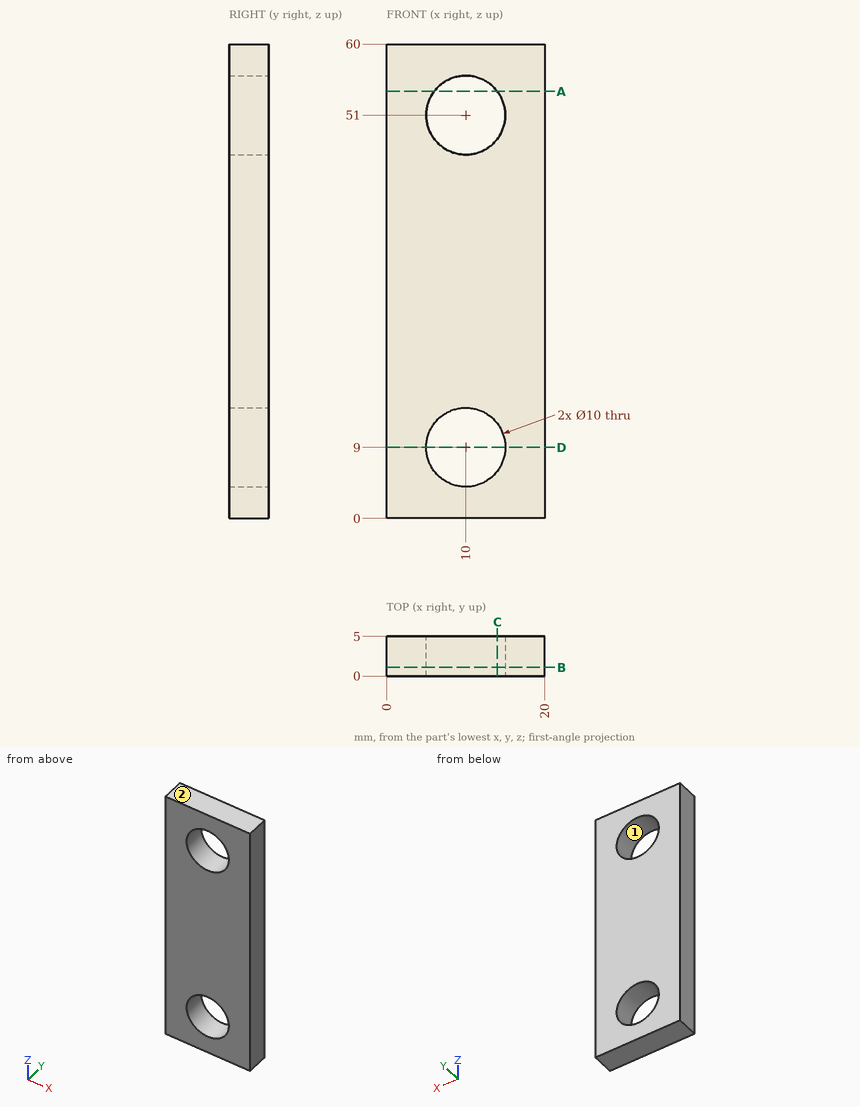
Here's the drawing with two shaded views (mm, measured from the low corner). I have some questions. Coordinates: 2 decimals unless noted, no trailing zeros. Loops run counter-clockwise (first coordinate to the right, second up) from the corner with the lowest first, then second, coordinate; pieces in that order, holes last. Notation, with made-up numbers: (38.5, 36) -> (95.5, 36) arc R23 cw to (95.5, 53) -> close; hole circle Ø6 at (0, -4.5). An arc over 180 degrees is marked (long way). Answer as a JSON object with one key per item and string values.
1) If I drill on line 1 (Z direction, x = 9.75, y = 0.7); line 2 (X direction, y = 2.45, z = 51); line 3 (Z direction, x = 7.75, y = 4.4), over which ranges is the centre line in solid material (lowest first)?
Results:
{"line 1": "z = 0 to 4.01, 13.99 to 46.01, 55.99 to 60", "line 2": "x = 0 to 5, 15 to 20", "line 3": "z = 0 to 4.53, 13.47 to 46.53, 55.47 to 60"}
2) Imagine slicing it at D-D (z = 9). Please give me the cut outline in (x, y).
Results:
{"outline": "(0, 0) -> (5, 0) -> (5, 5) -> (0, 5) -> close; (15, 0) -> (20, 0) -> (20, 5) -> (15, 5) -> close"}
3) Imagine slicing it at A-A (z = 54). Please give me the cut outline in (x, y).
Results:
{"outline": "(0, 0) -> (6, 0) -> (6, 5) -> (0, 5) -> close; (14, 0) -> (20, 0) -> (20, 5) -> (14, 5) -> close"}
4) Imagine slicing it at C-C (x = 14). Please give me the cut outline in (y, z), then the cut area to 3 significant figures.
Results:
{"outline": "(0, 0) -> (5, 0) -> (5, 6) -> (0, 6) -> close; (0, 12) -> (5, 12) -> (5, 48) -> (0, 48) -> close; (0, 54) -> (5, 54) -> (5, 60) -> (0, 60) -> close", "area": "240 mm^2"}
5) Imagine slicing it at B-B (y = 1.1). Please give me the cut outline in (x, z), then the cut area to 3 significant figures.
Results:
{"outline": "(0, 0) -> (20, 0) -> (20, 60) -> (0, 60) -> close; hole circle Ø10 at (10, 9); hole circle Ø10 at (10, 51)", "area": "1,040 mm^2"}
6) Thinking about a two-plate mould opening in X: for the marked faces 1 and 2, which applies, pulls with the +X half, pulls with the -X half, needs draft (parallel to the pull), parting line crosses it, or undercut?
Results:
{"face 1": "undercut", "face 2": "needs draft"}
